Check sheet for the modelled part. Datum: model origin and axes. Units: mm. Face numbers are marked on the shaded views. A direction names the side the tool comes from. Give positions to 0.01 mm unless a question says otherwise; leave off trailing zeros. Loops run counter-clockwise (first coordinate to the right, second up) from the corner with the lowest first, then second, coordinate; pieces in that order, holes last. Notation, with made-up numbers: M -25,80 L -17,80 A3 cw -17,84 Z; hole C 83,13.5 d1. An arc over 180 degrees is marked long. Use one line per item in the form item = value.
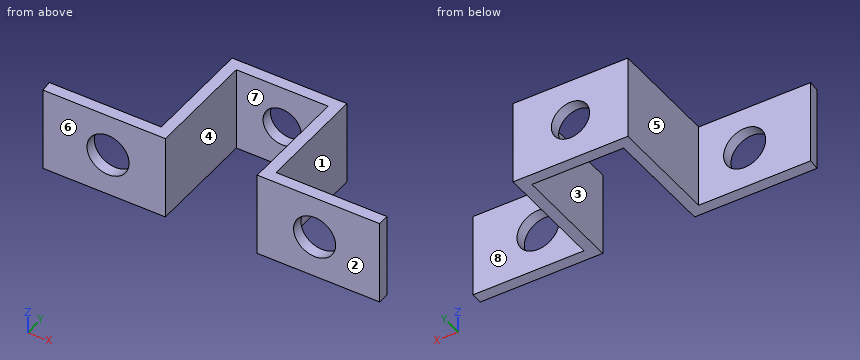
from build123d import *

# Parameters (mm, degrees)
F1_DEPTH = 22
F2_R     = 5
F3_DEPTH = 10
F4_R     = 5.5
F5_DEPTH = 25


# Not quite as in the source:
# - a feature names something its author has since deleted; it is built from what else it names


with BuildPart() as f1:
    # F0 (on Top) → F1 (new body)
    with BuildSketch(Plane.XY):
        Polygon((-15, -15.631636476), (-44.2782626623, -15.631636476), (-44, -18.631636476), (-12, -18.631636476), (-12, 10.368363524), (12, 10.368363524), (12, -18.631636476), (44, -18.631636476), (44, -15.631636476), (15, -15.631636476), (15, 13.368363524), (-15, 13.368363524), align=None)
    extrude(amount=F1_DEPTH)

    # F2 (on face) → F3 (cut)
    with BuildSketch(Plane(origin=(0, 13.368363524, 0), x_dir=(-1, 0, 0), z_dir=(0, 1, 0))):
        with Locations((0, 11)):
            Circle(F2_R)
    extrude(amount=-F3_DEPTH, mode=Mode.SUBTRACT)

    # F4 (on Front) → F5 (cut)
    with BuildSketch(Plane.XZ):
        with Locations((27, 11)):
            Circle(F4_R)
        with Locations((-27, 11)):
            Circle(F4_R)
    extrude(amount=F5_DEPTH, mode=Mode.SUBTRACT)


solid = f1.part
1) Section check D-D (z = 18.5). Record the cut outline in (x, y).
Evaluation:
outline = M -44.28,-15.63 L -44,-18.63 L -12,-18.63 L -12,10.37 L 12,10.37 L 12,-18.63 L 44,-18.63 L 44,-15.63 L 15,-15.63 L 15,13.37 L -15,13.37 L -15,-15.63 Z
2) Release check for a two-part mould opening along X. For the marked faces 1, 2, 3 and 4 record: pulls with the +X half, pulls with the -X half, needs draft (parallel to the pull), parting line crosses it, or undercut.
Evaluation:
face_1 = pulls with the +X half
face_2 = needs draft
face_3 = undercut
face_4 = undercut
3) Set-up check for the marked faces 5, 6, 7 and 8: record each of +Z, -Z, +X, -X, +Y, -Y from which the full face is reachable in a straight line by a thin tool's end or side.
Evaluation:
face_5 = +Z, -Z, -X, +Y
face_6 = +Z, -Z, +X, -X, -Y
face_7 = +Z, -Z, -Y
face_8 = +Z, -Z, +X, +Y
4) Section check B-B (y = -7.5). Record the cut outline in (x, z), then the cut area to 3 significant figures.
Evaluation:
outline = M -15,0 L -12,0 L -12,22 L -15,22 Z; M 12,0 L 15,0 L 15,22 L 12,22 Z
area = 132 mm^2
5) Depth check by flat-ended pin: pin 1 Ø6.5 at (x, z) = (-5, 6.5) entering from -Y; pin 2 Ø11 at (y, z) = (2, 5.5) entering from +X; pin 3 Ø6 at (y, z) = (-2.5, 19) entering from -X. Enter the tip coordinate at first touch or a pass-through.
Evaluation:
pin_1 = 10.37
pin_2 = 15
pin_3 = -15
6) Section check A-A (x = -27). Record the cut outline in (y, z).
Evaluation:
outline = M -18.63,0 L -15.63,0 L -15.63,5.5 L -18.63,5.5 Z; M -18.63,16.5 L -15.63,16.5 L -15.63,22 L -18.63,22 Z
7) Section check C-C (z = 11). Record the cut outline in (x, y), then the cut area to 3 significant figures.
Evaluation:
outline = M -44.28,-15.63 L -44,-18.63 L -32.5,-18.63 L -32.5,-15.63 Z; M -21.5,-18.63 L -12,-18.63 L -12,10.37 L -5,10.37 L -5,13.37 L -15,13.37 L -15,-15.63 L -21.5,-15.63 Z; M 5,10.37 L 12,10.37 L 12,-18.63 L 21.5,-18.63 L 21.5,-15.63 L 15,-15.63 L 15,13.37 L 5,13.37 Z; M 32.5,-18.63 L 44,-18.63 L 44,-15.63 L 32.5,-15.63 Z
area = 342 mm^2
8) Scan lines: line 1 (Z direction, x = 0, y = 11.2); line 2 (X direction, y = 9.5, z = 11); line 3 (Z direction, x = 27, y = -17). Record each from-to range of solid material in increasing order.
Evaluation:
line_1 = 0 to 6, 16 to 22
line_2 = -15 to -12, 12 to 15
line_3 = 0 to 5.5, 16.5 to 22
